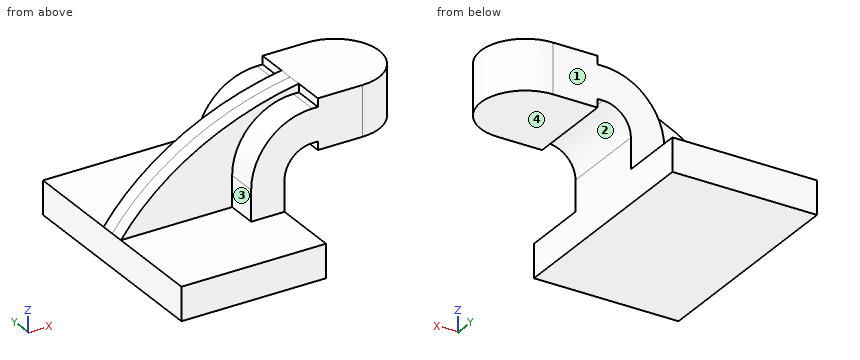
```python
from build123d import *

# Parameters (mm, degrees)
F1_DEPTH = 63.5
F2_DEPTH = 25.4
F3_DEPTH = 7.9375
F0_W     = 25.4
F0_H     = 28.575


with BuildPart() as f1:
    # F0 (on Front) → F1 (new body, symmetric)
    with BuildSketch(Plane.XZ):
        Polygon((-41.275, 9.525), (-41.275, -9.525), (41.275, -9.525), (41.275, 9.525), (22.225, 9.525), align=None)
    extrude(amount=F1_DEPTH, both=True)

    # F0 (on Front) → F2 (join, symmetric)
    with BuildSketch(Plane.XZ):
        with BuildLine():
            Line((22.225, 9.525), (41.275, 9.525))
            Line((41.275, 9.525), (41.275, 27.0002))
            ThreePointArc((41.275, 27.0002), (45.92468, 38.22552), (57.15, 42.8752))
            Line((57.15, 42.8752), (60.325, 42.8752))
            Line((60.325, 42.8752), (60.325, 61.9252))
            Line((60.325, 61.9252), (57.15, 61.9252))
            ThreePointArc((57.15, 61.9252), (32.454296, 51.695904), (22.225, 27.0002))
            Line((22.225, 27.0002), (22.225, 9.525))
        make_face()
        Polygon((85.725, 66.675), (60.325, 66.675), (60.325, 61.9252), (60.325, 42.8752), (60.325, 38.1), (85.725, 38.1), align=None)
    extrude(amount=F2_DEPTH, both=True)

    # F0 (on Front) → F3 (join, symmetric)
    with BuildSketch(Plane.XZ):
        with BuildLine():
            add(Edge.make_bspline(
                [(-41.275, 9.525), (-19.730542, 38.604709), (17.001747, 59.660653), (60.325, 66.675)],
                knots=[0, 0, 0, 0, 116.570504, 116.570504, 116.570504, 116.570504], degree=3))
            Line((-41.275, 9.525), (22.225, 9.525))
            Line((22.225, 9.525), (22.225, 27.0002))
            ThreePointArc((22.225, 27.0002), (32.454296, 51.695904), (57.15, 61.9252))
            Line((57.15, 61.9252), (60.325, 61.9252))
            Line((60.325, 61.9252), (60.325, 66.675))
        make_face()
    extrude(amount=F3_DEPTH, both=True)

    # F0 (on Front) → F4 (revolve)
    with BuildSketch(Plane.XZ):
        with Locations((98.425, 52.3875)):
            Rectangle(F0_W, F0_H)
    revolve(axis=Axis((85.725, 0, 52.3875), (0, 0, -1)))


solid = f1.part
```
Geometry: final body of the model. Coordinates: model frame, mm. Face numbers are marked on the shaded views. A direction names the side the tool comes from. Round coordinates to 2 decimals unless told otherwise and drop trailing zeros. Order: outer loops, then holes, each group sorted by start corner. A loop starts at its lowest first (then second) coordinate and runs counter-clockwise, first axis right, second up. Notation, with made-up numbers: (23, 42.25) - (60, 42.25) arc R10 ccw to (60, 47.25) - close; hole circle Ø2 at (-25, 49.5). An arc over 180 degrees is marked (long way). Write item = value, one per line. Start each with the question number.
Q1. Pin query (flat end, axial travel): pin 1 (5 mm diameter, centred on y = -16.5, z = 64.5, fed in from -X) (3 decimals); pin 2 (8 mm diameter, centred on x = 0, y = 12.5, fed in from +Z) (3 decimals); pin 3 (2 mm diameter, centred on y = -24, z = 35, fed in from +X). Return the tip coordinate at first contact, or that it passes through.
Q2. Ray query, line 1 (Z direction, x = 87, y = 17) (3 decimals); line 2 (Y direction, x = -2, z = 42.5); line 3 (Z direction, x = -12, y = -12) (3 decimals). Return the intervals inside material, ascending. Write a range as from..to.
Q3. Access query for the marked faces 1, 2, 3 and 4. Directions: +Z, -Z, +X, -X, +Y, -Y. A direction counts if a zero-diameter tool reaches every point of the face in a straight line with its end or side. Return the directions, or none.
Q4. Cut plane A-A on y = -13.5. Return the cut outline in (x, z) (3 decimals), and give its area (3 significant figures).
Q5. Cut plane B-B on y = -29. Return the cut outline in (x, z) (3 decimals).
Outcome:
q1.pin_1 = 60.325
q1.pin_2 = 9.525
q1.pin_3 = 44.07
q2.line_1 = 38.1..66.675
q2.line_2 = -7.94..7.94
q2.line_3 = -9.525..9.525
q3.face_1 = +Z, +X, -X, +Y
q3.face_2 = -Z, +Y, -Y
q3.face_3 = +Z, -X, -Y
q3.face_4 = -Z, +X, +Y, -Y
q4.outline = (-41.275, -9.525) - (41.275, -9.525) - (41.275, 27) arc R15.875 cw to (57.15, 42.875) - (60.325, 42.875) - (60.325, 38.1) - (107.24, 38.1) - (107.24, 66.675) - (60.325, 66.675) - (60.325, 61.925) - (57.15, 61.925) arc R34.925 ccw to (22.225, 27) - (22.225, 9.525) - (-41.275, 9.525) - close
q4.area = 4,070 mm^2
q5.outline = (-41.275, -9.525) - (41.275, -9.525) - (41.275, 9.525) - (-41.275, 9.525) - close
